from build123d import *

# Parameters (mm, degrees)
BASE_FLANGE1_DEPTH = 25
SKETCH6_R          = 6
CUT_EXTRUDE1_DEPTH = 10


# Sheet-metal steps are written as plain solids
with BuildPart() as part:
    # Sketch1 → Base-Flange1 (new body)
    with BuildSketch(Plane.XY):
        with BuildLine():
            Line((-57, 0), (-29, 0))
            ThreePointArc((-29, 0), (-25.173165676, 0.761204675), (-21.928932188, 2.928932188))
            Line((-21.928932188, 2.928932188), (-21.786796564, 3.071067812))
            ThreePointArc((-21.786796564, 3.071067812), (-18.542563076, 5.238795325), (-14.715728753, 6))
            Line((-14.715728753, 6), (14.715728753, 6))
            ThreePointArc((14.715728753, 6), (18.542563076, 5.238795325), (21.786796564, 3.071067812))
            Line((21.786796564, 3.071067812), (21.928932188, 2.928932188))
            ThreePointArc((21.928932188, 2.928932188), (25.173165676, 0.761204675), (29, 0))
            Line((29, 0), (57, 0))
            Line((57, 0), (57, -5))
            Line((57, -5), (29, -5))
            ThreePointArc((29, -5), (23.259748515, -3.858192988), (18.393398282, -0.606601718))
            Line((18.393398282, -0.606601718), (18.251262658, -0.464466094))
            ThreePointArc((18.251262658, -0.464466094), (16.629145914, 0.619397663), (14.715728753, 1))
            Line((14.715728753, 1), (-14.715728753, 1))
            ThreePointArc((-14.715728753, 1), (-16.629145914, 0.619397663), (-18.251262658, -0.464466094))
            Line((-18.251262658, -0.464466094), (-18.393398282, -0.606601718))
            ThreePointArc((-18.393398282, -0.606601718), (-23.259748515, -3.858192988), (-29, -5))
            Line((-29, -5), (-57, -5))
            Line((-57, -5), (-57, 0))
        make_face()
    extrude(amount=BASE_FLANGE1_DEPTH)

    # Sketch6 → Cut-Extrude1 (cut)
    with BuildSketch(Plane(origin=(0, 0, 0), x_dir=(1, 0, 0), z_dir=(0, 1, 0))):
        with BuildLine():
            ThreePointArc((-44.5, -25), (-53.338834765, -21.338834765), (-57, -12.5))
            Line((-57, -12.5), (-57, -25))
            Line((-57, -25), (-44.5, -25))
        make_face()
        with BuildLine():
            Line((-44.5, 0), (-57, 0))
            Line((-57, 0), (-57, -12.5))
            ThreePointArc((-57, -12.5), (-53.338834765, -3.661165235), (-44.5, 0))
        make_face()
        with Locations(Location((-44.5, -12.5, 0), (0, 0, 270))):
            Circle(SKETCH6_R)
        with Locations(Location((44.5, -12.5, 0), (0, 0, 270))):
            Circle(SKETCH6_R)
        with BuildLine():
            ThreePointArc((44.5, 0), (53.338834765, -3.661165235), (57, -12.5))
            Line((57, -12.5), (57, 0))
            Line((57, 0), (44.5, 0))
        make_face()
        with BuildLine():
            Line((44.5, -25), (57, -25))
            Line((57, -25), (57, -12.5))
            ThreePointArc((57, -12.5), (53.338834765, -21.338834765), (44.5, -25))
        make_face()
    extrude(amount=-CUT_EXTRUDE1_DEPTH, mode=Mode.SUBTRACT)


solid = part.part
The model under review builds one solid part; all positions refer to its coordinate system, in mm. A direction names the side the tool comes from. Round coordinates to 2 decimals unless told otherwise and drop trailing zeros. Loops run counter-clockwise (first coordinate to the right, second up) from the corner with the lowest first, then second, coordinate; pieces in that order, holes last. Notation, with made-up numbers: M 71.25,63 L 82.25,63 A16 ccw 82.25,79 Z; hole C -0.75,19 d11. An arc over 180 degrees is marked long. Answer as CSV lines item,"result".
1. We need section A-A (y = -2). Give the boundary of the cut face in (x, z).
Outcome:
outline,"M -44.5,0 L -20,0 L -20,25 L -44.5,25 A12.5 ccw Z; M 20,0 L 44.5,0 A12.5 ccw 44.5,25 L 20,25 Z; hole C -44.5,12.5 d12; hole C 44.5,12.5 d12"
2. We need section D-D (x = 36.5). Give the boundary of the cut face in (y, z).
Outcome:
outline,"M -5,0 L 0,0 L 0,25 L -5,25 Z"
3. We need section B-B (z = 13.5). Give the boundary of the cut face in (x, y).
Outcome:
outline,"M -56.96,-5 L -50.42,-5 L -50.42,0 L -56.96,0 Z; M -38.58,-5 L -29,-5 A15 ccw -18.39,-0.61 L -18.25,-0.46 A5 cw -14.72,1 L 14.72,1 A5 cw 18.25,-0.46 L 18.39,-0.61 A15 ccw 29,-5 L 38.58,-5 L 38.58,0 L 29,0 A10 cw 21.93,2.93 L 21.79,3.07 A10 ccw 14.72,6 L -14.72,6 A10 ccw -21.79,3.07 L -21.93,2.93 A10 cw -29,0 L -38.58,0 Z; M 50.42,-5 L 56.96,-5 L 56.96,0 L 50.42,0 Z"
4. To check wall thickness, follow L1, parallel to X at y = -3.15, z = 12.5; L2, parallel to X at y = -3.5, z = 7.5; L3, parallel to Y at x = -0.5, z = 21. State the ranges of each line that lie inside material, in increasing order. Write a range as [from, to].
Outcome:
L1,"x = [-57, -50.5], [-38.5, -21.78], [21.78, 38.5], [50.5, 57]"
L2,"x = [-55.96, -47.82], [-41.18, -22.46], [22.46, 41.18], [47.82, 55.96]"
L3,"y = [1, 6]"
5. Insertion check: pin 1 Ø12.5 at (x, z) = (-7, 10.5) entering from -Y; pin 2 Ø7.5 at (x, z) = (48, 7.5) entering from +Y; pin 3 Ø8 at (x, z) = (-21.5, 17) entering from -Y. Each pin has a flat end and moves straight along its axis. Give the tip position at first contact, or say it passes through.
Outcome:
pin 1,"stops at y = 1"
pin 2,"stops at y = 0"
pin 3,"stops at y = -4.59"
6. For faces 1 (the face through (-37, 0, 12)), 2 (the face through (16.65, 0.61, 12.32)), 3 (the face through (37, 0, 12)), list the 3-axis set-ups (+Z, -Z, +X, -X, +Y, -Y) from which the entire face can be reached by the end or side of a thin tool; tool diameter is ignored.
Outcome:
face 1,"+Z, -Z, -X, +Y"
face 2,"+Z, -Z, -Y"
face 3,"+Z, -Z, +X, +Y"
7. We need section C-C (z = 2). Give the boundary of the cut face in (x, y), plus the area to 3 significant figures.
Outcome:
outline,"M -51.28,-5 L -29,-5 A15 ccw -18.39,-0.61 L -18.25,-0.46 A5 cw -14.72,1 L 14.72,1 A5 cw 18.25,-0.46 L 18.39,-0.61 A15 ccw 29,-5 L 51.28,-5 L 51.28,0 L 29,0 A10 cw 21.93,2.93 L 21.79,3.07 A10 ccw 14.72,6 L -14.72,6 A10 ccw -21.79,3.07 L -21.93,2.93 A10 cw -29,0 L -51.28,0 Z"
area,"529 mm2"
8. Draft analysis for pull direction X (two halves, no side actions). For faces 4 (the face through (1, 2, 25)), 5 (the face through (-16.6, 0.63, 12.32)), 6 (the face through (25.122, 0.782, 12.325)), state which applies: pulls with the +X half, pulls with the -X half, needs draft (parallel to the pull), parting line crosses it, or undercut.
Outcome:
face 4,"needs draft"
face 5,"undercut"
face 6,"pulls with the +X half"
